Read the model definition and answer for the solid it produces. Units are mm, in the model's axes. Face numbers are marked on the shaded views. A direction names the side the tool comes from. Give positions to 0.01 mm unless a question says otherwise; leave off trailing zeros. Loops run counter-clockwise (first coordinate to the right, second up) from the corner with the lowest first, then second, coordinate; pieces in that order, holes last. Notation, with made-up numbers: (-19.5, 30.5) -> (-4.5, 30.5) arc R27 ccw to (-4.5, 62.5) -> close; hole circle Ø8 at (37.5, 72). An arc over 180 degrees is marked (long way). Write each question's results on one line, items separated by ' | '. Start each with the question number.
Item 1: Determine the mould class of the marked faces 1, 2 and 3 for opening direction Y: +Y half, -Y half, draft (parallel to the pull), parting line (faces both ways), or undercut.
Item 2: Find the intervals of material crossed by line 1 (X direction, y = -40, z = 2.25); line 2 (Y direction, x = 15.5, z = 4.75); line 3 (Y direction, x = 40, z = 8), in increasing order.
Item 3: Section B-B on z = 8 is taken. Write down the section's boundary in (x, y), and give its area (3 significant figures).
Item 4: Section A-A on y = -16 is taken. Write down the section's boundary in (x, z), and give its area (3 significant figures).
Item 5: Section C-C on x = 38.5 is taken. Write down the section's boundary in (y, z), and give its area (3 significant figures).
Item 6: Which of the six approach directions +Z, -Z, +X, -X, +Y, -Y give full straight-line access (tool end or side, diameter ignored) to the marked faces 4, 5 and 6?
Item 7: Each of these flat-tipped pins is pushed along its axis until it touches: P1, Ø3, axis at x = 35.5, z = 2, coming from the -Y side; P2, Ø4, axis at x = 28, z = 5, coming from the -Y side. Where does it stop, or does it pass through?
```python
from build123d import *

# Parameters (mm, degrees)
BOSS_EXTRUDE1_DEPTH = 12.7


with BuildPart() as part:
    # Sketch2 → Boss-Extrude1 (new body)
    with BuildSketch(Plane.XY):
        with BuildLine():
            Line((0, 0), (49.530251281, 0))
            Line((49.530251281, 0), (49.530251281, -59.689999999))
            ThreePointArc((49.530251281, -59.689999999), (48.786302505, -61.486051224), (46.990251281, -62.229999999))
            Line((46.990251281, -62.229999999), (44.232383169, -62.229999999))
            ThreePointArc((44.232383169, -62.229999999), (43.260344035, -62.036644396), (42.436296408, -61.486015686))
            Line((42.436296408, -61.486015686), (36.830502562, -55.879999999))
            Line((36.830502562, -55.879999999), (40.640502562, -55.879999999))
            ThreePointArc((40.640502562, -55.879999999), (42.436553786, -55.136051224), (43.180502562, -53.339999999))
            Line((43.180502562, -53.339999999), (43.180502562, -6.35))
            Line((43.180502562, -6.35), (0, -6.35))
            Line((0, -6.35), (0, -53.339999999))
            ThreePointArc((0, -53.339999999), (0.743948776, -55.136051224), (2.54, -55.879999999))
            Line((2.54, -55.879999999), (6.35, -55.879999999))
            Line((6.35, -55.879999999), (0.744206153, -61.486015686))
            ThreePointArc((0.744206153, -61.486015686), (-0.079841474, -62.036644396), (-1.051880608, -62.229999999))
            Line((-1.051880608, -62.229999999), (-3.809748719, -62.229999999))
            ThreePointArc((-3.809748719, -62.229999999), (-5.605799943, -61.486051224), (-6.349748719, -59.689999999))
            Line((-6.349748719, -59.689999999), (-6.349748719, 0))
            Line((-6.349748719, 0), (0, 0))
        make_face()
    extrude(amount=BOSS_EXTRUDE1_DEPTH)


solid = part.part
```
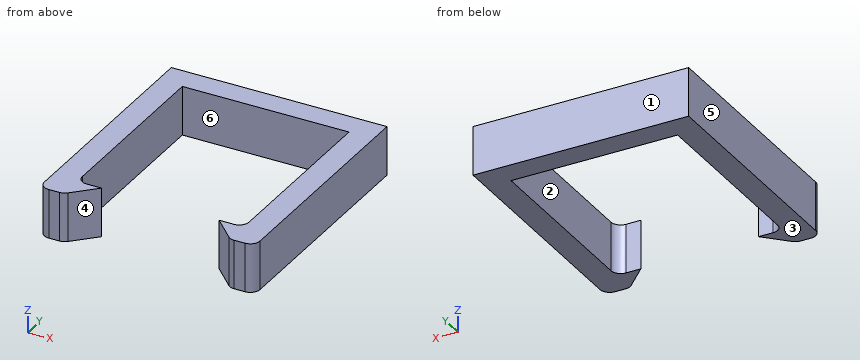
Findings:
1) face 1: +Y half | face 2: undercut | face 3: draft
2) line 1: -6.35 to 0, 43.18 to 49.53 | line 2: -6.35 to 0 | line 3: -59.05 to -55.88, -6.35 to 0
3) outline: (-6.35, -59.69) arc R2.54 ccw to (-3.81, -62.23) -> (-1.05, -62.23) arc R2.54 ccw to (0.74, -61.49) -> (6.35, -55.88) -> (2.54, -55.88) arc R2.54 cw to (0, -53.34) -> (0, -6.35) -> (43.18, -6.35) -> (43.18, -53.34) arc R2.54 cw to (40.64, -55.88) -> (36.83, -55.88) -> (42.44, -61.49) arc R2.54 ccw to (44.23, -62.23) -> (46.99, -62.23) arc R2.54 ccw to (49.53, -59.69) -> (49.53, 0) -> (-6.35, 0) -> close | area: 1,100 mm2
4) outline: (-6.35, 0) -> (0, 0) -> (0, 12.7) -> (-6.35, 12.7) -> close; (43.18, 0) -> (49.53, 0) -> (49.53, 12.7) -> (43.18, 12.7) -> close | area: 161 mm2
5) outline: (-57.55, 0) -> (-55.88, 0) -> (-55.88, 12.7) -> (-57.55, 12.7) -> close; (-6.35, 0) -> (0, 0) -> (0, 12.7) -> (-6.35, 12.7) -> close | area: 102 mm2
6) face 4: +Z, -Z, -Y | face 5: +Z, -Z, -X, +Y, -Y | face 6: +Z, -Z
7) P1: y = -56.05 | P2: y = -6.35
